```python
from build123d import *

# Parameters (mm, degrees)
SKETCH1_R           = 32.385
BOSS_EXTRUDE1_DEPTH = 2
FILLET1_R           = 6.35
SKETCH2_R           = 2.2225
CUT_EXTRUDE1_DEPTH  = 52.017498224
SKETCH5_R           = 0.762
CUT_EXTRUDE2_DEPTH  = 52.017498224


with BuildPart() as part:
    # Sketch1 → Boss-Extrude1 (new body)
    with BuildSketch(Plane(origin=(0, 0, 0), x_dir=(1, 0, 0), z_dir=(0, 1, 0))):
        Circle(SKETCH1_R)
        with BuildLine():
            Line((-27.94, 27.737218678), (-27.94, 16.375122137))
            ThreePointArc((-27.94, 16.375122137), (0, 32.385), (27.94, 16.375122137))
            Line((27.94, 16.375122137), (27.94, 27.737218678))
            ThreePointArc((27.94, 27.737218678), (0, 39.37), (-27.94, 27.737218678))
        make_face()
    extrude(amount=BOSS_EXTRUDE1_DEPTH)

    # Fillet1
    fillet1_edges = [part.edges().sort_by_distance(p)[0] for p in [
        (-27.94, 1, -27.737218678),
        (27.94, 1, -27.737218678),
    ]]
    fillet(fillet1_edges, radius=FILLET1_R)

    # Sketch2 → Cut-Extrude1 (cut, through all)
    with BuildSketch(Plane(origin=(0, 2, 0), x_dir=(1, 0, 0), z_dir=(0, 1, 0))):
        with Locations(Location((0, 34.544, 0), (0, 0, 270))):
            Circle(SKETCH2_R)
    extrude(amount=-CUT_EXTRUDE1_DEPTH, mode=Mode.SUBTRACT)

    # Sketch5 → Cut-Extrude2 (cut, through all)
    with BuildSketch(Plane(origin=(0, 2, 0), x_dir=(1, 0, 0), z_dir=(0, 1, 0))):
        with Locations(Location((9.8425, 10.2235, 0), (0, 0, 270))):
            Circle(SKETCH5_R)
        with Locations(Location((12.3825, 10.2235, 0), (0, 0, 270))):
            Circle(SKETCH5_R)
        with Locations(Location((14.9225, 10.2235, 0), (0, 0, 270))):
            Circle(SKETCH5_R)
        with Locations(Location((17.4625, 10.2235, 0), (0, 0, 270))):
            Circle(SKETCH5_R)
        with Locations(Location((9.8425, 7.6835, 0), (0, 0, 270))):
            Circle(SKETCH5_R)
        with Locations(Location((12.3825, 7.6835, 0), (0, 0, 270))):
            Circle(SKETCH5_R)
        with Locations(Location((14.9225, 7.6835, 0), (0, 0, 270))):
            Circle(SKETCH5_R)
        with Locations(Location((17.4625, 7.6835, 0), (0, 0, 270))):
            Circle(SKETCH5_R)
        with Locations(Location((9.8425, 5.1435, 0), (0, 0, 270))):
            Circle(SKETCH5_R)
        with Locations(Location((12.3825, 5.1435, 0), (0, 0, 270))):
            Circle(SKETCH5_R)
        with Locations(Location((14.9225, 5.1435, 0), (0, 0, 270))):
            Circle(SKETCH5_R)
        with Locations(Location((17.4625, 5.1435, 0), (0, 0, 270))):
            Circle(SKETCH5_R)
        with Locations(Location((9.8425, 2.6035, 0), (0, 0, 270))):
            Circle(SKETCH5_R)
        with Locations(Location((12.3825, 2.6035, 0), (0, 0, 270))):
            Circle(SKETCH5_R)
        with Locations(Location((14.9225, 2.6035, 0), (0, 0, 270))):
            Circle(SKETCH5_R)
        with Locations(Location((17.4625, 2.6035, 0), (0, 0, 270))):
            Circle(SKETCH5_R)
        with Locations(Location((9.8425, 0.0635, 0), (0, 0, 270))):
            Circle(SKETCH5_R)
        with Locations(Location((12.3825, 0.0635, 0), (0, 0, 270))):
            Circle(SKETCH5_R)
        with Locations(Location((14.9225, 0.0635, 0), (0, 0, 270))):
            Circle(SKETCH5_R)
        with Locations(Location((17.4625, 0.0635, 0), (0, 0, 270))):
            Circle(SKETCH5_R)
    extrude(amount=-CUT_EXTRUDE2_DEPTH, mode=Mode.SUBTRACT)


solid = part.part
```
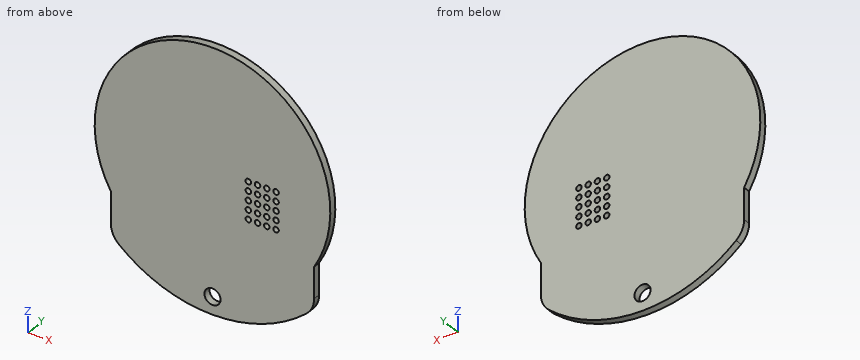
Source: CAD feature listing. Evaluate the final solid. Frame: model axes, mm. Coordinates: 2 decimals unless noted, no trailing zeros. Loops run counter-clockwise (first coordinate to the right, second up) from the corner with the lowest first, then second, coordinate; pieces in that order, holes last. Notation, with made-up numbers: (67, 1.5) - (80, 1.5) arc R27 ccw to (80, 20.5) - close; hole circle Ø4 at (37, -28.5). An arc over 180 degrees is marked (long way). Answer as CSV lines item,"result".
1. Section B-B (y = 1.1). Count the separate pieces of the cut face and the enclosed holes in it, then the cut area to 3 significant figures.
Established:
separate pieces,"1"
enclosed holes,"21"
area,"3,690 mm2"
2. Ray query, line 1 (Z direction, x = 15, y = 1.1); line 2 (X direction, y = 0.95, z = -8); line 3 (Z direction, x = 10, y = 0.6). Return the intervals inside material, ascending.
Established:
line 1,"z = -36.4 to -10.98, -9.47 to -8.44, -6.93 to -5.9, -4.39 to -3.36, -1.85 to -0.82, 0.69 to 28.7"
line 2,"x = -31.38 to 9.15, 10.54 to 11.69, 13.08 to 14.23, 15.62 to 16.77, 18.16 to 31.38"
line 3,"z = -38.08 to -10.97, -9.48 to -8.43, -6.94 to -5.89, -4.4 to -3.35, -1.86 to -0.81, 0.68 to 30.8"
3. Section A-A (x = 0). Return loops of the section in (y, z) (1 decimal).
Established:
outline,"(0, -39.4) - (2, -39.4) - (2, -36.8) - (0, -36.8) - close; (0, -32.3) - (2, -32.3) - (2, 32.4) - (0, 32.4) - close"
4. Contact query for a flat-ended pin moving along its axis: pin 1 (1 mm diameter, centred on y = 1, z = -21, fed in from +X). Output: stop coordinate, or through.
Established:
pin 1,"stops at x = 27.94"
5. Section C-C (z = 26.5). Return loops of the section in (x, y).
Established:
outline,"(-18.62, 0) - (18.62, 0) - (18.62, 2) - (-18.62, 2) - close"
6. Section D-D (x = 7). Return loops of the section in (y, z).
Established:
outline,"(0, -38.74) - (2, -38.74) - (2, 31.62) - (0, 31.62) - close"
